Geometry: final body of the model. Coordinates: model frame, mm. Give positions to 0.01 mm unless a question says otherwise; leave off trailing zeros. Write each loop counter-clockwise with the first axis right and the second up, starting at its lowest first coordinate (ties: lowest second). Pieces come first, ordered by that corner, then holes. Notation, with made-up numbers: M 84.25,24.25 L 118.25,24.25 A26 cw 118.25,42.25 Z; hole C 83.5,6.5 d8. An arc over 180 degrees is marked long. Use a Markdown table: item, result. Add a question column.
1) Pin query (flat end, axial travel): pin 1 (0.6 mm diameter, centred on x = 0, y = 0, fed in from -Z). Return the tip coordinate at first contact, or that it passes through.
2) Section B-B on x = 0. Return the cut outline in (y, z) (3 decimals), then the cut area to 3 significant figures.
3) Section C-C on z = 84. Return the cut outline in (x, y) (3 decimals), then the cut area to 3 significant figures.
4) Line query: line 1 (X direction, y = -0.45, z = 114.5). Output: solid intervals per line, ascending.
5) Section A-A on y = 0. Return the cut outline in (x, z) (3 decimals), then the cut area to 3 significant figures.
```python
from build123d import *

# Parameters (mm, degrees)
SKETCH1_R           = 0.635
SKETCH1_R_2         = 0.5334
BOSS_EXTRUDE1_DEPTH = 125
SKETCH2_W           = 0.7
SKETCH2_H           = 0.8668
CUT_EXTRUDE1_DEPTH  = 25


with BuildPart() as part:
    # Sketch1 → Boss-Extrude1 (new body)
    with BuildSketch(Plane.XY):
        Circle(SKETCH1_R)
        Circle(SKETCH1_R_2, mode=Mode.SUBTRACT)
    extrude(amount=BOSS_EXTRUDE1_DEPTH)

    # Sketch2 → Cut-Extrude1 (cut)
    with BuildSketch(Plane.XY):
        with Locations((0, 0.5334)):
            Rectangle(SKETCH2_W, SKETCH2_H)
    extrude(amount=CUT_EXTRUDE1_DEPTH, mode=Mode.SUBTRACT)


solid = part.part
```
Found:
| question | item | result |
|---|---|---|
| 1 | pin 1 | through |
| 2 | outline | M -0.635,0 L -0.533,0 L -0.533,125 L -0.635,125 Z; M 0.533,25 L 0.635,25 L 0.635,125 L 0.533,125 Z |
| 2 | area | 22.9 mm² |
| 3 | outline | C 0,0 d1.27; hole C 0,0 d1.067 |
| 3 | area | 0.373 mm² |
| 4 | line 1 | -0.45 to -0.29, 0.29 to 0.45 |
| 5 | outline | M -0.635,0 L -0.533,0 L -0.533,125 L -0.635,125 Z; M 0.533,0 L 0.635,0 L 0.635,125 L 0.533,125 Z |
| 5 | area | 25.4 mm² |
